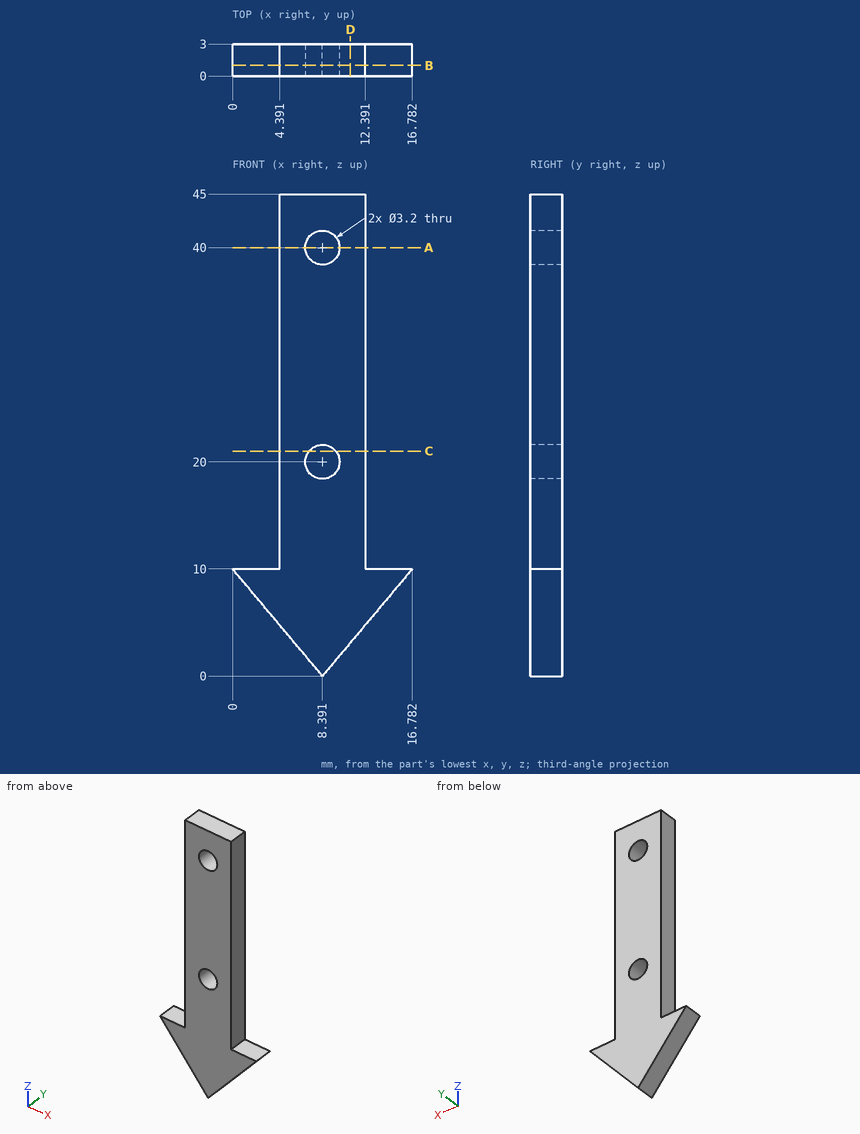
The drawing under review shows one solid part. Ordinate dimensions are in mm from its lowest x, y, z. Give positions to 0.01 mm unless a question says otherwise; leave off trailing zeros. Write each loop counter-clockwise with the first axis right and the second up, starting at its lowest first coordinate (ties: lowest second). Pieces come first, ordered by that corner, then holes.
1. Add section A-A, the plane z = 40. Write out the cut boundary in (x, y).
2. Add section C-C, the plane z = 21. Write out the cut boundary in (x, y).
3. For P1, Ø5, axis at x = 8.39, z = 40, coming from the +Y side; P2, Ø0.9, axis at x = 15, y = 1.5, coming from the +Z side, all flat-tipped, find the tip position at first contact; note any pin that passes through.
4. Add section D-D, the plane x = 11. Write out the cut boundary in (y, z), plus the area to 3 significant figures.
5. Wall thickness on L1, parallel to Z at x = 8, y = 1.1; L2, parallel to X at y = 1, z = 20; L3, parallel to Z at x = 9.75, y = 0.4: over which ranges is each line inside the solid? List them lowest first.
6. Add section B-B, the plane y = 1. Write out the cut boundary in (x, z).
Worked answers:
1. outline: (4.39, 0) - (6.79, 0) - (6.79, 3) - (4.39, 3) - close; (9.99, 0) - (12.39, 0) - (12.39, 3) - (9.99, 3) - close
2. outline: (4.39, 0) - (7.14, 0) - (7.14, 3) - (4.39, 3) - close; (9.64, 0) - (12.39, 0) - (12.39, 3) - (9.64, 3) - close
3. P1: stops at y = 3
3. P2: stops at z = 10
4. outline: (0, 3.11) - (3, 3.11) - (3, 45) - (0, 45) - close
4. area: 126 mm2
5. L1: z = 0.47 to 18.45, 21.55 to 38.45, 41.55 to 45
5. L2: x = 4.39 to 6.79, 9.99 to 12.39
5. L3: z = 1.62 to 19.16, 20.84 to 39.16, 40.84 to 45
6. outline: (0, 10) - (8.39, 0) - (16.78, 10) - (12.39, 10) - (12.39, 45) - (4.39, 45) - (4.39, 10) - close; hole circle Ø3.2 at (8.39, 20); hole circle Ø3.2 at (8.39, 40)
